The listing builds one solid part. Answer for the finished solid, in the listing's coordinates (mm). A direction names the side the tool comes from. Coordinates: 2 decimals unless noted, no trailing zeros. Order: outer loops, then holes, each group sorted by start corner. A loop starts at its lowest first (then second) coordinate and runs counter-clockwise, first axis right, second up. Notation, with made-up numbers: (13.5, 20) -> (17.5, 20) arc R11 cw to (17.5, 36) -> close; hole circle Ø1 at (70.25, 15). An arc over 180 degrees is marked (long way). Write each question's results on one line, items separated by ' | '. Start each with the question number.
(1) The part is cut by section A-A, the plane x = 4.5. Give the vertices of the cut face in (y, z).
(2) The part is cut by section D-D, the plane z = 5.5. Give the vertices of the cut face in (x, y).
(3) A tool of negligible diameter and unlimited length cuts with its end or side. For faces 4 (the face through (32, 41.9, 9)), 5 (the face through (52.5, 33, 2)), 6 (the face through (12.27, 14.2, 0.76)), 7 (the face through (11.95, 51.12, 0.76)), 8 (the face through (14.5, 30, 9)), from which of +Z, -Z, +X, -X, +Y, -Y can it reach the whole face along a straight path? Write none if from no direction.
(4) Given pin 1 (3.5 mm diameter, centred on y = 38, z = 3, fed in from -X); pin 2 (7 mm diameter, centred on x = 17, y = 52, fed in from +Z); pin 3 (5.5 mm diameter, centred on x = 60.5, y = 12.5, fed in from -Z); pin 4 (7 mm diameter, centred on y = 25.5, z = 7.5, fed in from +X), each flat-ended and moving along its own axis, determine where each tip first touches the part or whether it passes through.
(5) Straight lines are drawn through the part: L1, parallel to X at y = 30.5, z = 8.25; L2, parallel to Y at x = 15, z = 0.4; L3, parallel to X at y = 31, z = 3.25. For each, find the intervals that lie inside material, in ascending order.
(6) Determine the mould class of faces 1 (the face through (12.5, 33, 2)), 2 (the face through (32, 34, 0)), 3 (the face through (57.618, 19.759, 0.76)) for opening direction Y: +Y half, -Y half, draft (parallel to the pull), parting line (faces both ways), or undercut.
(7) The part is cut by section C-C, the plane x = 21. Give the vertices of the cut face in (y, z).
(8) The part is cut by section B-B, the plane y = 35. Give the vertices of the cut face in (x, z), then the cut area to 3 significant figures.
```python
from build123d import *
from build123d import SkipClean  # not in build123d's __all__

# Parameters (mm, degrees)
F0_R     = 1.65
F1_DEPTH = 1.5
F3_DEPTH = 1.501
F4_DEPTH = 1.5
F5_W     = 40
F5_H     = 30
F6_DEPTH = 3
F7_W     = 36
F7_H     = 23.3
F8_DEPTH = 9


with BuildPart() as f1:
    # F0 (on Top) → F1 (new body)
    with BuildSketch(Plane.XY):
        with BuildLine():
            ThreePointArc((-0.73370891, 14), (-0.4891889552, 6.9935887205), (0, 0))
            Line((0, 0), (65, 0))
            ThreePointArc((65, 0), (65.4891889552, 6.9935887205), (65.73370891, 14))
            ThreePointArc((65.73370891, 14), (65.7334108185, 21.0021379582), (65.488741818, 28))
            Line((65.488741818, 28), (57.299411547, 50.5))
            ThreePointArc((57.299411547, 50.5), (32.5, 63.5), (7.700588453, 50.5))
            Line((7.700588453, 50.5), (-0.488741818, 28))
            ThreePointArc((-0.488741818, 28), (-0.7334108185, 21.0021379582), (-0.73370891, 14))
        make_face()
        with Locations((4.5, 12.5)):
            Circle(F0_R, mode=Mode.SUBTRACT)
        with Locations((60.5, 12.5)):
            Circle(F0_R, mode=Mode.SUBTRACT)
        with Locations((15, 54.5)):
            Circle(F0_R, mode=Mode.SUBTRACT)
    extrude(amount=F1_DEPTH)

    # F2 (on face) → F3 (cut, through all)
    with BuildSketch(Plane.XY.offset(1.5)):
        with BuildLine():
            ThreePointArc((15.3946260476, 58.178895253), (17.4713893755, 57.2535857631), (18.6149922575, 55.2885626028))
            Line((18.6149922575, 55.2885626028), (20.0740134556, 48.6))
            Line((20.0740134556, 48.6), (52.5, 48.6))
            Line((52.5, 48.6), (52.5, 24.064025175))
            Line((52.5, 24.064025175), (62.8817094627, 15.3315119698))
            ThreePointArc((62.8817094627, 15.3315119698), (63.8542752579, 14.0616777817), (64.2, 12.5))
            ThreePointArc((64.2, 12.5), (62.0616777817, 9.1457247421), (58.1182905373, 9.6684880302))
            Line((58.1182905373, 9.6684880302), (47.5, 18.6))
            Line((47.5, 18.6), (17.5, 18.6))
            Line((17.5, 18.6), (6.8817094627, 9.6684880302))
            ThreePointArc((6.8817094627, 9.6684880302), (1.6684880302, 10.1182905373), (2.1182905373, 15.3315119698))
            Line((2.1182905373, 15.3315119698), (12.5, 24.064025175))
            Line((12.5, 24.064025175), (12.5, 48.6))
            Line((12.5, 48.6), (11.3850077425, 53.7114373972))
            ThreePointArc((11.3850077425, 53.7114373972), (11.308192582, 54.2539146721), (11.3123280961, 54.8017878876))
            ThreePointArc((11.3123280961, 54.8017878876), (9.4060764304, 52.7351735725), (7.700588453, 50.5))
            Line((7.700588453, 50.5), (-0.488741818, 28))
            ThreePointArc((-0.488741818, 28), (-0.733560046, 13.9914611719), (0, 0))
            Line((0, 0), (65, 0))
            ThreePointArc((65, 0), (65.733560046, 13.9914611719), (65.488741818, 28))
            Line((65.488741818, 28), (57.299411547, 50.5))
            ThreePointArc((57.299411547, 50.5), (37.9351551683, 63.0061258111), (15.3946260476, 58.178895253))
        make_face()
    extrude(amount=-F3_DEPTH, mode=Mode.SUBTRACT)

    # F2 (on face) → F4 (join)
    with BuildSketch(Plane.XY.offset(1.5)):
        with BuildLine():
            ThreePointArc((11.3123280961, 54.8017878876), (13.2791635515, 56.5801728664), (15.3946260476, 58.178895253))
            ThreePointArc((15.3946260476, 58.178895253), (12.6415574435, 57.3509206772), (11.3123280961, 54.8017878876))
        make_face()
    with SkipClean():  # cleaning this boolean's faces spoils the solid; the shape is the same uncleaned
        extrude(amount=-F4_DEPTH)

    # F5 (on face) → F6 (join)
    with BuildSketch(Plane.XY.offset(1.5)):
        with Locations((32.5, 33.6)):
            Rectangle(F5_W, F5_H)
    extrude(amount=F6_DEPTH)

    # F7 (on face) → F8 (join)
    with BuildSketch(Plane.XY.offset(4.5)):
        with Locations((32.5, 30.25)):
            Rectangle(F7_W, F7_H)
    extrude(amount=F8_DEPTH)


solid = f1.part
```
Established:
1) outline: (8.8, 0) -> (10.85, 0) -> (10.85, 1.5) -> (8.8, 1.5) -> close; (14.15, 0) -> (17.33, 0) -> (17.33, 1.5) -> (14.15, 1.5) -> close
2) outline: (14.5, 18.6) -> (50.5, 18.6) -> (50.5, 41.9) -> (14.5, 41.9) -> close
3) face 4: +Z, +X, -X, +Y | face 5: +Z, +X, +Y | face 6: +Z, -Z, -Y | face 7: +Z, -Z, -X | face 8: +Z, -X, +Y, -Y
4) pin 1: stops at x = 12.5 | pin 2: stops at z = 4.5 | pin 3: stops at z = 0 | pin 4: stops at x = 52.5
5) L1: x = 14.5 to 50.5 | L2: y = 16.5 to 52.85, 56.15 to 58.2 | L3: x = 12.5 to 52.5
6) face 1: undercut | face 2: draft | face 3: +Y half
7) outline: (18.6, 0) -> (48.6, 0) -> (48.6, 4.5) -> (41.9, 4.5) -> (41.9, 13.5) -> (18.6, 13.5) -> close
8) outline: (12.5, 0) -> (52.5, 0) -> (52.5, 4.5) -> (50.5, 4.5) -> (50.5, 13.5) -> (14.5, 13.5) -> (14.5, 4.5) -> (12.5, 4.5) -> close | area: 504 mm^2
